```python
from build123d import *

# Parameters (mm, degrees)
PAD_DEPTH = 10
FILLET_R  = 2.99


with BuildPart() as part:
    # Sketch → Pad (new body)
    with BuildSketch(Plane.XY):
        with BuildLine():
            ThreePointArc((5, -11.456439), (5.06017, 11.42999), (-11.842719, -4))
            Line((-11.842719, -4), (-17.527225, -5.92))
            ThreePointArc((11, -14.874475), (5.540471, 17.650869), (-17.527225, -5.92))
            Line((11, -14.874475), (11, -28.117345))
            ThreePointArc((-16.970563, -36.365151), (5.09102, -59.630189), (11, -28.117345))
            Line((-11.313708, -38.365151), (-16.970563, -36.365151))
            ThreePointArc((-11.313708, -38.365151), (4.679562, -53.415115), (5, -31.456439))
            Line((5, -11.456439), (5, -31.456439))
        make_face()
    extrude(amount=PAD_DEPTH)

    # Fillet
    fillet_edges = [part.edges().sort_by_distance(p)[0] for p in [
        (-17.527225, -5.92, 5),
        (-11.842719, -4, 5),
        (-11.313708, -38.365151, 5),
        (-16.970563, -36.365151, 5),
        (5, -31.456439, 5),
        (5, -11.456439, 5),
        (11, -14.874475, 5),
        (11, -28.117345, 5),
    ]]
    fillet(fillet_edges, radius=FILLET_R)


solid = part.part
```
Verification items for the finished model (mm, model axes). A direction names the side the tool comes from. Round coordinates to 2 decimals unless told otherwise and drop trailing zeros. Loops run counter-clockwise (first coordinate to the right, second up) from the corner with the lowest first, then second, coordinate; pieces in that order, holes last. Notation, with made-up numbers: (-28, 20) -> (18, 20) arc R13 cw to (18, 41) -> close; hole circle Ø4 at (58.5, 26.25). An arc over 180 degrees is marked (long way). Answer as a JSON object with one key per item and string values.
Q1. Scan lines: line 1 (Y direction, x = 0, z = 6.75); line 2 (X direction, y = 0, z = 6); line 3 (Y direction, x = 6.5, z = 2.5). Record each from-to range of solid material in increasing order. Write a range as from..to.
Data:
{"line 1": "y = -60.37..-54.37, 12.5..18.5", "line 2": "x = -18.5..-12.5, 12.5..18.5", "line 3": "y = -59.15..-52.45, -32.28..-10.68, 10.68..17.32"}
Q2. Section check B-B (y = 5). Record the boundary of the cut face in (x, z), then the cut area to 3 significant figures.
Data:
{"outline": "(-17.81, 0) -> (-11.46, 0) -> (-11.46, 10) -> (-17.81, 10) -> close; (11.46, 0) -> (17.81, 0) -> (17.81, 10) -> (11.46, 10) -> close", "area": "127 mm2"}
Q3. Access from +Z, -Z, +X, -X, +Y, -Y to the whole of each face (thin tool, end or side, straight path). Record for faces 5 (the cylindrical face through (-12.803, -3.586, 5.07)), 6 (the flat face through (11, -21, 5)), 7 (the cylindrical face through (5.383, -31.145, 5.07)).
Data:
{"face 5": "+Z, -Z", "face 6": "+Z, -Z, +X", "face 7": "+Z, -Z, -X"}
Q4. Go/stop test with flat-tipped pins: P1, Ø5, axis at x = -5.5, z = 2, coming from the +Y side; P2, Ø20, axis at x = 0, y = 0, coming from the -Z side; P3, Ø1.5, axis at y = -34.5, z = 4, coming from the +X side. Record where each tip stops, or that it passes through.
Data:
{"P1": "stops at y = 18.26", "P2": "passes through", "P3": "stops at x = 16.53"}
Q5. Draft check along X on faces 1 (the cylindrical face through (-16.448, -37.745, 5.07)), 2 (the cylindrical face through (7.102, 17.082, 4.93)), 3 (the cylindrical face through (11.254, -27.922, 5.07)), 4 (the flat face through (7, -24, 0)). Enter one of: pulls with the +X half, pulls with the -X half, needs draft (parallel to the pull), parting line crosses it, or undercut.
Data:
{"face 1": "undercut", "face 2": "parting line crosses it", "face 3": "pulls with the +X half", "face 4": "needs draft"}
Q6. Section check C-C (x = 8). Record the boundary of the cut face in (y, z), then the cut area to 3 significant figures.
Data:
{"outline": "(-58.49, 0) -> (-51.31, 0) -> (-51.31, 10) -> (-58.49, 10) -> close; (-33.42, 0) -> (-9.6, 0) -> (-9.6, 10) -> (-33.42, 10) -> close; (9.6, 0) -> (16.68, 0) -> (16.68, 10) -> (9.6, 10) -> close", "area": "381 mm2"}
Q7. Section check A-A (x = 0). Record the boundary of the cut face in (y, z).
Data:
{"outline": "(-60.37, 0) -> (-54.37, 0) -> (-54.37, 10) -> (-60.37, 10) -> close; (12.5, 0) -> (18.5, 0) -> (18.5, 10) -> (12.5, 10) -> close"}
